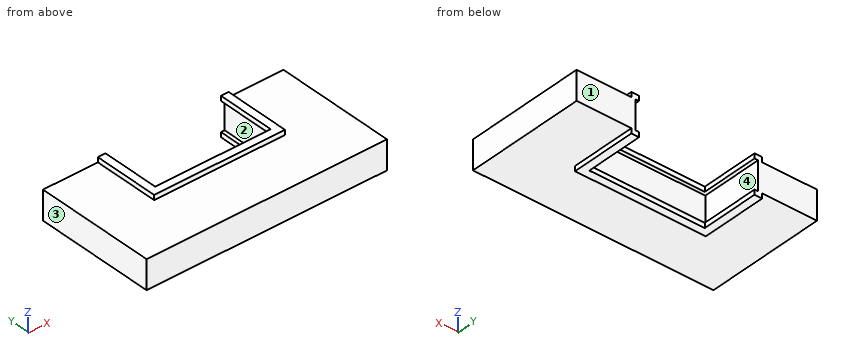
```python
from build123d import *

# Parameters (mm, degrees)
SKETCH1_W           = 25
SKETCH1_H           = 12.5
BOSS_EXTRUDE1_DEPTH = 3
BOSS_EXTRUDE3_START = -1.5
SKETCH2_W           = 13.6
SKETCH2_H           = 6.8
BOSS_EXTRUDE3_DEPTH = 2
CUT_EXTRUDE2_START  = -2
SKETCH4_W           = 12.75
SKETCH4_H           = 6.375
CUT_EXTRUDE2_DEPTH  = 1.5
SKETCH5_W           = 12
SKETCH5_H           = 6
CUT_EXTRUDE3_DEPTH  = 5


with BuildPart() as part:
    # Sketch1 → Boss-Extrude1 (new body)
    with BuildSketch(Plane.XY):
        Rectangle(SKETCH1_W, SKETCH1_H)
    extrude(amount=BOSS_EXTRUDE1_DEPTH)

    # Sketch2 → Boss-Extrude3 (add, symmetric)
    with BuildSketch(Plane.XY.offset(3).offset(BOSS_EXTRUDE3_START)):
        with Locations((0, 2.85)):
            Rectangle(SKETCH2_W, SKETCH2_H)
    extrude(amount=BOSS_EXTRUDE3_DEPTH, both=True)

    # Sketch4 → Cut-Extrude2 (cut, symmetric)
    with BuildSketch(Plane.XY.offset(3.5).offset(CUT_EXTRUDE2_START)):
        with Locations((0, 3.0625)):
            Rectangle(SKETCH4_W, SKETCH4_H)
    extrude(amount=CUT_EXTRUDE2_DEPTH, both=True, mode=Mode.SUBTRACT)

    # Sketch5 → Cut-Extrude3 (cut)
    with BuildSketch(Plane.XY.offset(3.5)):
        with Locations((0, 3.25)):
            Rectangle(SKETCH5_W, SKETCH5_H)
    extrude(amount=-CUT_EXTRUDE3_DEPTH, mode=Mode.SUBTRACT)


solid = part.part
```
Geometry: final body of the model. Coordinates: model frame, mm. Face numbers are marked on the shaded views. A direction names the side the tool comes from. Coordinates: 2 decimals unless noted, no trailing zeros. Order: outer loops, then holes, each group sorted by start corner. A loop starts at its lowest first (then second) coordinate and runs counter-clockwise, first axis right, second up. Notation, with made-up numbers: (19, -40) -> (64, -40) arc R13 cw to (64, -17) -> close; hole circle Ø2 at (89.25, -21). An arc over 180 degrees is marked (long way). Use CSV: the item, a comma, the result in double quotes.
1) Pin query (flat end, axial travel): pin 1 Ø0.6 at (y, z) = (4, -0.5) entering from +X; pin 2 Ø5 at (x, y) = (0, 3.5) entering from -Z; pin 3 Ø0.9 at (x, z) = (-2, 2) entering from +Y (3 decimals). Return the tip coordinate at first contact, or that it passes through.
Findings:
pin 1,"stops at x = 6.8"
pin 2,"passes through"
pin 3,"stops at y = -0.125"
2) Mould query, pull axis Z, two halves, no side actions, for the marked faces 3 and 4. Classes: +Z half, -Z half, draft (parallel to the pull), parting line (faces both ways), or undercut.
Findings:
face 3,"draft"
face 4,"undercut"
3) Access query for the marked faces 1 and 2. Directions: +Z, -Z, +X, -X, +Y, -Y. A direction counts if a zero-diameter tool reaches every point of the face in a straight line with its end or side. Return the directions, or none.
Findings:
face 1,"+Z, -Z, +X, -X, +Y"
face 2,"+Y"
4) Section A-A on y = 5.25. Output: boundary loops of the cut face in (x, z) (3 decimals), then the cut area to 4 significant figures.
Findings:
outline,"(-12.5, 0) -> (-6.8, 0) -> (-6.8, -0.5) -> (-6, -0.5) -> (-6, 0) -> (-6.375, 0) -> (-6.375, 3) -> (-6, 3) -> (-6, 3.5) -> (-6.8, 3.5) -> (-6.8, 3) -> (-12.5, 3) -> close; (6, -0.5) -> (6.8, -0.5) -> (6.8, 0) -> (12.5, 0) -> (12.5, 3) -> (6.8, 3) -> (6.8, 3.5) -> (6, 3.5) -> (6, 3) -> (6.375, 3) -> (6.375, 0) -> (6, 0) -> close"
area,"38.35 mm^2"
5) Line query: line 1 (X direction, y = 0.5, z = 2.95) (3 decimals); line 2 (Z direction, x = 3.25, y = 0); line 3 (Y direction, x = -2, z = 0.3) (3 decimals). Output: solid intervals per line, ascending.
Findings:
line 1,"x = -12.5 to -6.375, 6.375 to 12.5"
line 2,"z = -0.5 to 0, 3 to 3.5"
line 3,"y = -6.25 to -0.125"
6) Section C-C on x = 0.75. Output: boundary loops of the cut face in (y, z) (3 decimals).
Findings:
outline,"(-6.25, 0) -> (-0.55, 0) -> (-0.55, -0.5) -> (0.25, -0.5) -> (0.25, 0) -> (-0.125, 0) -> (-0.125, 3) -> (0.25, 3) -> (0.25, 3.5) -> (-0.55, 3.5) -> (-0.55, 3) -> (-6.25, 3) -> close"
7) Section B-B on z = 2.15. Output: boundary loops of the cut face in (x, y) (3 decimals), then the cut area to 3 significant figures.
Findings:
outline,"(-12.5, -6.25) -> (12.5, -6.25) -> (12.5, 6.25) -> (6.375, 6.25) -> (6.375, -0.125) -> (-6.375, -0.125) -> (-6.375, 6.25) -> (-12.5, 6.25) -> close"
area,"231 mm^2"
8) Section D-D on y = -3.5. Output: boundary loops of the cut face in (x, z), then the cut area to 3 significant figures.
Findings:
outline,"(-12.5, 0) -> (12.5, 0) -> (12.5, 3) -> (-12.5, 3) -> close"
area,"75.0 mm^2"
